Here's how the part is built. I have some questions about the finished solid (model axes, mm). Face numbers are marked on the shaded views. Round coordinates to 2 decimals unless told otherwise and drop trailing zeros. Write each loop counter-clockwise with the first axis right and the second up, starting at its lowest first coordinate (ties: lowest second). Pieces come first, ordered by that corner, then holes. Notation, with made-up numbers: (26.5, 71.5) -> (36.5, 71.5) arc R20 ccw to (36.5, 108.5) -> close; hole circle Ø10 at (-35.5, 74.5). An arc over 180 degrees is marked (long way). Put each result on its own line as item: value. Start each with the question number.
1. Suppose I cut it at C-C (z = -6.5). Please give me the cut outline in (x, y).
2. Suppose I cut it at A-A (y = 0). Please give me the cut outline in (x, z).
3. I need wall thicknesses on probe 1 along Y at (x, z) = (11, -5.75); probe 2 along X at (y, z) = (1.5, -7.5); probe 3 along X at (y, z) = (-4.5, -6). Which ranges of each line are inside material? Lowest first, please. Write a range as from..to.
4. For pin 1 (4 mm diameter, centred on x = 19, z = -6.35, fed in from +Y) (3 decimals), with a flat end and sliding along its axis, tell me the tip position at first contact or that it passes through.
5. We'd pull the mould along X, two halves only. Please class the marked faces 1, 2, 3 and 4: +X half, -X half, draft (parallel to the pull), parting line (faces both ways), or undercut.
6. Suppose I cut it at B-B (x = 3). Please give me the cut outline in (y, z).
7. Suppose I cut it at D-D (y = 3.5). Please give me the cut outline in (x, z), then the cut area to 3 significant figures.
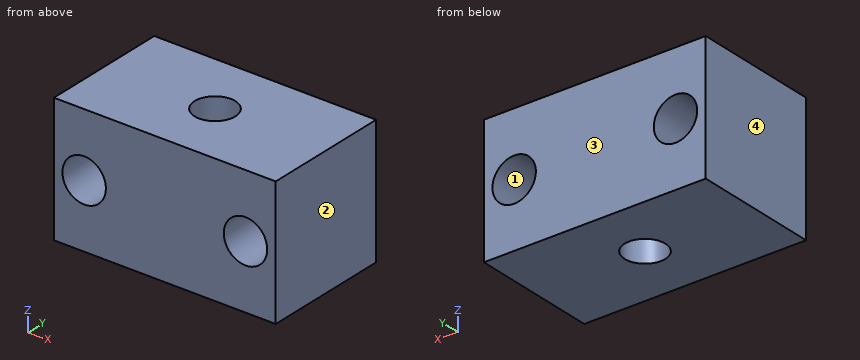
```python
from build123d import *

# Parameters (mm, degrees)
SKETCH1_W                    = 22.000000004
SKETCH1_H                    = 12.7
BOSS_EXTRUDE1_DEPTH          = 6.35
F_18_0_1695_DIAMETER_HOLE1_D = 4.3053
F_18_0_1695_DIAMETER_HOLE2_D = 4.3053
F_10_32_TAPPED_HOLE1_D       = 4.0386


with BuildPart() as part:
    # Sketch1 → Boss-Extrude1 (new, symmetric)
    with BuildSketch(Plane(origin=(0, 0, 0), x_dir=(1, 0, 0), z_dir=(0, 1, 0))):
        with Locations((11.000000002, 6.35)):
            Rectangle(SKETCH1_W, SKETCH1_H)
    extrude(amount=BOSS_EXTRUDE1_DEPTH, both=True)

    # #18 (0.1695) Diameter Hole1 (through all)
    with Locations(Plane(origin=(3, 6.35, -6.35), x_dir=(0, 0, 1), z_dir=(0, 1, 0))):
        with Locations((0, 0)):
            Hole(F_18_0_1695_DIAMETER_HOLE1_D / 2)

    # #18 (0.1695) Diameter Hole2 (through all)
    with Locations(Plane(origin=(19.000000004, 6.35, -6.35), x_dir=(0, 0, 1), z_dir=(0, 1, 0))):
        with Locations((0, 0)):
            Hole(F_18_0_1695_DIAMETER_HOLE2_D / 2)

    # #10-32 Tapped Hole1 (through all)
    with Locations(Plane(origin=(11.000000002, 0, -12.7), x_dir=(-1, 0, 0), z_dir=(0, 0, -1))):
        with Locations((0, 0)):
            Hole(F_10_32_TAPPED_HOLE1_D / 2)


solid = part.part
```
Verdict:
1. outline: (0, -6.35) -> (0.85, -6.35) -> (0.85, 6.35) -> (0, 6.35) -> close; (5.15, -6.35) -> (16.85, -6.35) -> (16.85, 6.35) -> (5.15, 6.35) -> close; (21.15, -6.35) -> (22, -6.35) -> (22, 6.35) -> (21.15, 6.35) -> close; hole circle Ø4.04 at (11, 0)
2. outline: (0, -12.7) -> (8.98, -12.7) -> (8.98, 0) -> (0, 0) -> close; (13.02, -12.7) -> (22, -12.7) -> (22, 0) -> (13.02, 0) -> close; hole circle Ø4.31 at (3, -6.35); hole circle Ø4.31 at (19, -6.35)
3. probe 1: y = -6.35..-2.02, 2.02..6.35
3. probe 2: x = 0..1.18, 4.82..9.65, 12.35..17.18, 20.82..22
3. probe 3: x = 0..0.88, 5.12..16.88, 21.12..22
4. pin 1: passes through
5. face 1: undercut
5. face 2: +X half
5. face 3: draft
5. face 4: -X half
6. outline: (-6.35, -12.7) -> (6.35, -12.7) -> (6.35, -8.5) -> (-6.35, -8.5) -> close; (-6.35, -4.2) -> (6.35, -4.2) -> (6.35, 0) -> (-6.35, 0) -> close
7. outline: (0, -12.7) -> (22, -12.7) -> (22, 0) -> (0, 0) -> close; hole circle Ø4.31 at (3, -6.35); hole circle Ø4.31 at (19, -6.35)
7. area: 250 mm^2
